Geometry: see drawing. Coordinates: mm, zero at the bounding-box minimum. Give positions to 0.01 mm unless a question says otherwise; leave off trailing zeros. Put each result on its own line as item: value. Start each with the question number.
1. Ray query, line 1 along Y through (x, z) = (25, 5); line 2 along Y through (x, z) = (16, 6.25) (1 decimal); line 3 along X through (y, z) = (40, 7.5). Return the intervals inside material, ascending. Write a range as from..to.
2. Section A-A on z = 13. Count the separate pieces of the cut face and the enclosed holes in it, plus the area to 3 significant figures.
3. Mould query, pull axis Y, two halves, no side actions, for the marked faces 1, 2 and 3. Classes: pulls with the +Y half, pulls with the -Y half, needs draft (parallel to the pull), parting line crosses it, or undercut.
4. First-contact query: P1, Ø5, axis at x = 44.5, z = 11.5, coming from the -Y side; P2, Ø2, axis at y = 19.5, z = 8, coming from the +X side; P3, Ø3, axis at y = 41, z = 7.5, coming from the +X side (1 decimal). Flat tips, straight axial feed; report the tip coordinate or a pass-through.
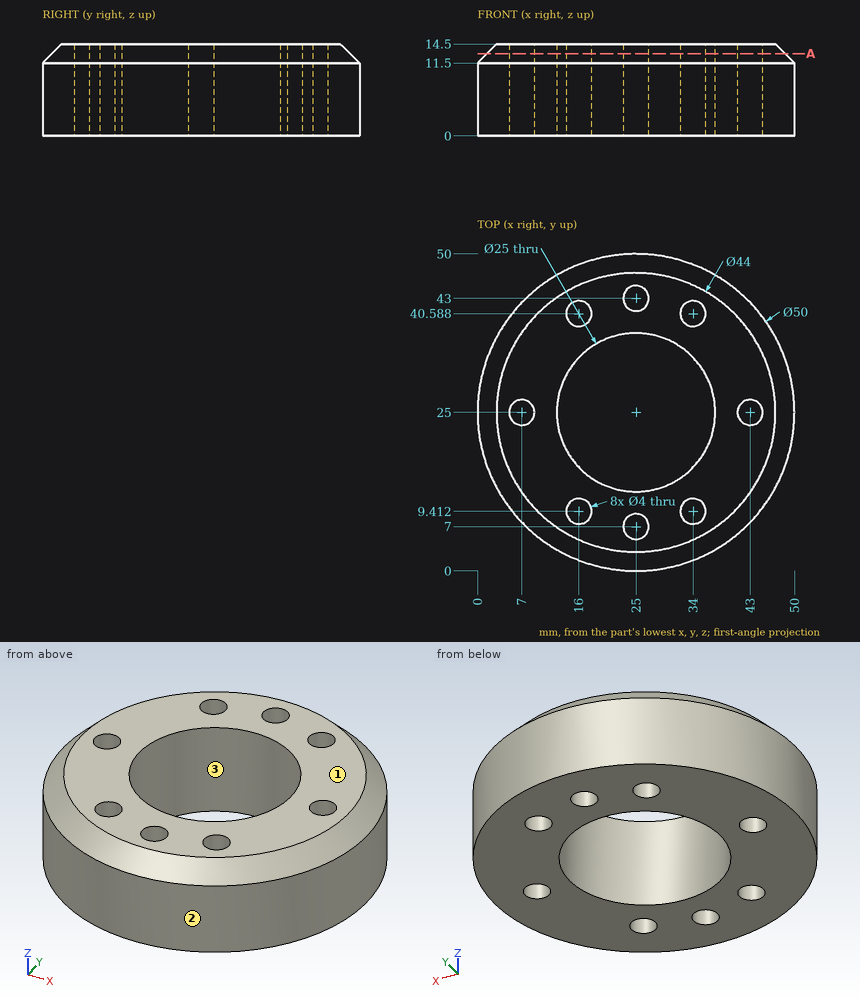
Resolved:
1. line 1: 0..5, 9..12.5, 37.5..41, 45..50
1. line 2: 1.7..7.4, 11.4..16.3, 33.7..38.6, 42.6..48.3
1. line 3: 5..14.09, 17.91..32.09, 35.91..45
2. separate pieces: 1
2. enclosed holes: 9
2. area: 1,140 mm^2
3. face 1: needs draft
3. face 2: parting line crosses it
3. face 3: undercut
4. P1: y = 6.67
4. P2: x = 49.59
4. P3: x = 45.4
